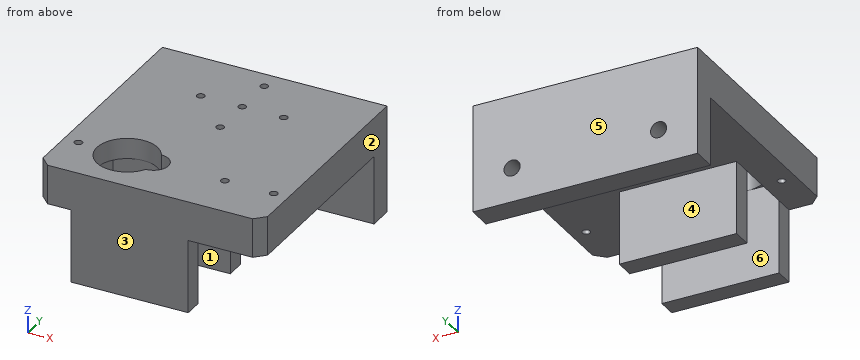
```python
from build123d import *

# Parameters (mm, degrees)
SKETCH_1_W                  = 46
SKETCH_1_H                  = 48
EXTRUDE_1_DEPTH             = 8
CHAMFER_1_SIZE              = 2
SKETCH_2_W                  = 46
SKETCH_2_H                  = 5
EXTRUDE_2_DEPTH             = 14
HOLE_WIZARD_M4_1_D          = 3.3
HOLE_WIZARD_M4_1_DEPTH      = 11.5
HOLE_WIZARD_M4_1_TIP        = 0.991420021
HOLE_WIZARD_M2_1_AT_2_COUNT = 2
HOLE_WIZARD_M2_1_AT_2_PITCH = 10
SKETCH_8_R                  = 0.8
CUT_EXTRUDE_1_DEPTH         = 23
SKETCH_9_W                  = 24
SKETCH_9_H                  = 12.4
CUT_EXTRUDE_2_DEPTH         = 3.8
SKETCH_11_W                 = 24
SKETCH_11_H                 = 3.8
SKETCH_11_H_2               = 4
EXTRUDE_3_DEPTH             = 15
FILLET_1_R                  = 3
HOLE_WIZARD_M2_2_D          = 1.6
HOLE_WIZARD_M2_2_DEPTH      = 5.2
HOLE_WIZARD_M2_2_TIP        = 0.480688495
HOLE_WIZARD_M2_3_D          = 1.6
HOLE_WIZARD_M2_3_DEPTH      = 5.2
HOLE_WIZARD_M2_3_TIP        = 0.480688495


with BuildPart() as part:
    # 草图1 → 凸台-拉伸1 (new body)
    with BuildSketch(Plane.XY):
        Rectangle(SKETCH_1_W, SKETCH_1_H)
    extrude(amount=EXTRUDE_1_DEPTH)

    # 倒角1
    chamfer_1_edges = [part.edges().sort_by_distance(p)[0] for p in [
        (23, -24, 4),
        (-23, -24, 4),
    ]]
    chamfer(chamfer_1_edges, length=CHAMFER_1_SIZE)

    # 草图2 → 凸台-拉伸2 (add)
    with BuildSketch(Plane(origin=(0, 0, 0), x_dir=(-1, 0, 0), z_dir=(0, 0, -1))):
        with Locations((0, 21.5)):
            Rectangle(SKETCH_2_W, SKETCH_2_H)
    extrude(amount=EXTRUDE_2_DEPTH)

    # M4 螺纹孔1
    with Locations(Plane(origin=(0, 24, 0), x_dir=(1, 0, 0), z_dir=(0, 1, 0))):
        with Locations((15, 7), (-15, 7)):
            Hole(HOLE_WIZARD_M4_1_D / 2, depth=HOLE_WIZARD_M4_1_DEPTH)
            with Locations((0, 0, -(HOLE_WIZARD_M4_1_DEPTH + HOLE_WIZARD_M4_1_TIP / 2))):  # 118° drill point
                Cone(0, HOLE_WIZARD_M4_1_D / 2, HOLE_WIZARD_M4_1_TIP, mode=Mode.SUBTRACT)

    # 草图6 → M2 螺纹孔1 (revolve, cut)
    with BuildSketch(Plane(origin=(10, -14, 8), x_dir=(0, -1, 0), z_dir=(1, 0, 0))):
        Polygon((0, 0), (0, 46.480688495), (0.8, 46), (0.8, 0), align=None)
    hole_wizard_m2_1 = revolve(axis=Axis((10, -14, 14.35), (0, 0, -1)), mode=Mode.SUBTRACT)

    # M2 螺纹孔1 at 2: M2 螺纹孔1 ×2
    with Locations(*[(i * HOLE_WIZARD_M2_1_AT_2_PITCH, 0, 0) for i in range(1, HOLE_WIZARD_M2_1_AT_2_COUNT)]):
        add(hole_wizard_m2_1, mode=Mode.SUBTRACT)

    # 镜向1: M2 螺纹孔1 across plane
    add(hole_wizard_m2_1.mirror(Plane(origin=(0, 0, 0), x_dir=(0, 0, 1), z_dir=(1, 0, 0))), mode=Mode.SUBTRACT)

    # 镜向1 copy 1 sketch → 镜向1 copy 1 (revolve, cut)
    with BuildSketch(Plane(origin=(-20, -14, 8), x_dir=(0, -1, 0), z_dir=(-1, 0, 0))):
        Polygon((0, 0), (0, -46.480688495), (0.8, -46), (0.8, 0), align=None)
    revolve(axis=Axis((-20, -14, 14.35), (0, 0, 1)), mode=Mode.SUBTRACT)

    # 草图8 → 切除-拉伸1 (cut)
    # profile 1 of 3: a face of its own
    with BuildSketch(Plane.XY.offset(8)):
        with BuildLine():
            ThreePointArc((-4.574136013, -11), (-16.2, -14), (-4.574136013, -17))
            Line((-4.574136013, -17), (-4.574136013, -11))
        make_face()
        with Locations((-10, -14)):
            Circle(SKETCH_8_R, mode=Mode.SUBTRACT)
    # profile 2 of 3: a face of its own
    with BuildSketch(Plane.XY.offset(8)):
        with BuildLine():
            Line((-4.574136013, -11), (-4.574136013, -17))
            ThreePointArc((-4.574136013, -17), (-3.996652737, -15.549135773), (-3.8, -14))
            ThreePointArc((-3.8, -14), (-3.996652737, -12.450864227), (-4.574136013, -11))
        make_face()
    # profile 3 of 3: a face of its own
    with BuildSketch(Plane.XY.offset(8)):
        with BuildLine():
            ThreePointArc((-3.8, -14), (-3.996652737, -15.549135773), (-4.574136013, -17))
            Line((-4.574136013, -17), (-1.574136013, -17))
            Line((-1.574136013, -17), (-1.574136013, -11))
            Line((-1.574136013, -11), (-4.574136013, -11))
            ThreePointArc((-4.574136013, -11), (-3.996652737, -12.450864227), (-3.8, -14))
        make_face()
    extrude(amount=-CUT_EXTRUDE_1_DEPTH, mode=Mode.SUBTRACT)

    # 草图9 → 切除-拉伸2 (cut)
    with BuildSketch(Plane(origin=(0, 0, 0), x_dir=(-1, 0, 0), z_dir=(0, 0, -1))):
        with Locations((4.2, -14)):
            Rectangle(SKETCH_9_W, SKETCH_9_H)
    extrude(amount=-CUT_EXTRUDE_2_DEPTH, mode=Mode.SUBTRACT)

    # 草图11 → 凸台-拉伸3 (add)
    with BuildSketch(Plane(origin=(0, 0, 0), x_dir=(-1, 0, 0), z_dir=(0, 0, -1))):
        with Locations((4.2, -22.1)):
            Rectangle(SKETCH_11_W, SKETCH_11_H)
        with Locations((4.2, -5.8)):
            Rectangle(SKETCH_11_W, SKETCH_11_H_2)
    extrude(amount=EXTRUDE_3_DEPTH)

    # 圆角1
    fillet_1_edges = [part.edges().sort_by_distance(p)[0] for p in [
        (-1.574136013, -11, 5.9),
        (-1.574136013, -17, 5.9),
    ]]
    fillet(fillet_1_edges, radius=FILLET_1_R - 0.0001)  # a hair under: the kernel refuses the full size

    # M2 螺纹孔2
    with Locations(Plane.XY.offset(8)):
        with Locations((0, 11.5)):
            Hole(HOLE_WIZARD_M2_2_D / 2, depth=HOLE_WIZARD_M2_2_DEPTH)
            with Locations((0, 0, -(HOLE_WIZARD_M2_2_DEPTH + HOLE_WIZARD_M2_2_TIP / 2))):  # 118° drill point
                Cone(0, HOLE_WIZARD_M2_2_D / 2, HOLE_WIZARD_M2_2_TIP, mode=Mode.SUBTRACT)

    # M2 螺纹孔3
    with Locations(Plane(origin=(0, 20, 8), x_dir=(1, 0, 0), z_dir=(0, 0, 1))):
        with Locations((0, 0), (8.5, -8.5), (0, -17), (-8.5, -8.5)):
            Hole(HOLE_WIZARD_M2_3_D / 2, depth=HOLE_WIZARD_M2_3_DEPTH)
            with Locations((0, 0, -(HOLE_WIZARD_M2_3_DEPTH + HOLE_WIZARD_M2_3_TIP / 2))):  # 118° drill point
                Cone(0, HOLE_WIZARD_M2_3_D / 2, HOLE_WIZARD_M2_3_TIP, mode=Mode.SUBTRACT)


solid = part.part
```
Check sheet for the modelled part. Datum: model origin and axes. Units: mm. Face numbers are marked on the shaded views. A direction names the side the tool comes from. Give positions to 0.01 mm unless a question says otherwise; leave off trailing zeros. Loops run counter-clockwise (first coordinate to the right, second up) from the corner with the lowest first, then second, coordinate; pieces in that order, holes last. Notation, with made-up numbers: (82.5, 12) - (140.5, 12) arc R30 ccw to (140.5, 51) - close; hole circle Ø1 at (14, 15). An arc over 180 degrees is marked (long way). One line per question, with ' | ' between items. Start each with the question number.
1. Cross-section at D-D, the plane x = -14.5. Enter the section's corners in (y, z), plus the area to 3 significant figures.
2. Cross-section at A-A, the plane z = -10. Enter the section's corners in (x, y).
3. Cross-section at B-B, the plane x = 15. Enter the section's corners in (y, z).
4. Material ranges on line 1 along Y through (x, z) = (4.5, -13); line 2 along Y through (x, z) = (0, 6.9); line 3 along X through (y, z) = (20.6, -7), recorded low to high. Write a range as [from, to].
5. Gauge pin test, flat ends, axial feed: pin 1 Ø2.5 at (x, y) = (8.5, 20.5) entering from -Z; pin 2 Ø2 at (y, z) = (-6.5, -10) entering from +X; pin 3 Ø6 at (x, y) = (2.5, -13.5) entering from -Z. Record the tip position at first contact, or that the pin passes through.
6. Cross-section at C-C, the plane z = 6.25. Give the number of separate pieces and of enclosed holes in the cut face, plus the area to 3 significant figures.
7. Draft check along X on the marked faces 1, 2 and 3. Enter one of: released by +X, released by -X, zero draft, split by the parting line, or undercut.
8. Set-up check for the marked faces 4, 5 and 6: record each of +Z, -Z, +X, -X, +Y, -Y from which the full face is reachable in a straight line by a thin tool's end or side.
Check result:
1) outline: (-24, -15) - (-20.2, -15) - (-20.2, 3.8) - (-18.26, 3.8) - (-18.26, 8) - (-24, 8) - close; (-9.74, 3.8) - (-7.8, 3.8) - (-7.8, -15) - (-3.8, -15) - (-3.8, 0) - (19, 0) - (19, -5.43) - (24, -5.43) - (24, 8) - (-9.74, 8) - close; (19, -14) - (24, -14) - (24, -8.57) - (19, -8.57) - close | area: 472 mm2
2) outline: (-23, 19) - (23, 19) - (23, 24) - (-23, 24) - close; (-16.2, -24) - (7.8, -24) - (7.8, -20.2) - (-16.2, -20.2) - close; (-16.2, -7.8) - (7.8, -7.8) - (7.8, -3.8) - (-16.2, -3.8) - close
3) outline: (-24, 0) - (19, 0) - (19, -5.35) - (24, -5.35) - (24, 8) - (-24, 8) - close; (19, -14) - (24, -14) - (24, -8.65) - (19, -8.65) - close
4) line 1: y = [-24, -20.2], [-7.8, -3.8], [19, 24] | line 2: y = [-24, 2.2], [3.8, 10.7], [12.3, 19.2], [20.8, 24] | line 3: x = [-23, -16.65], [-13.35, 13.35], [16.65, 23]
5) pin 1: stops at z = -14 | pin 2: stops at x = 7.8 | pin 3: stops at z = 3.8
6) separate pieces: 1 | enclosed holes: 9 | area: 2,060 mm2
7) face 1: undercut | face 2: released by +X | face 3: zero draft
8) face 4: -Z, +X, -X | face 5: +Z, -Z, +X, -X, +Y | face 6: -Z
